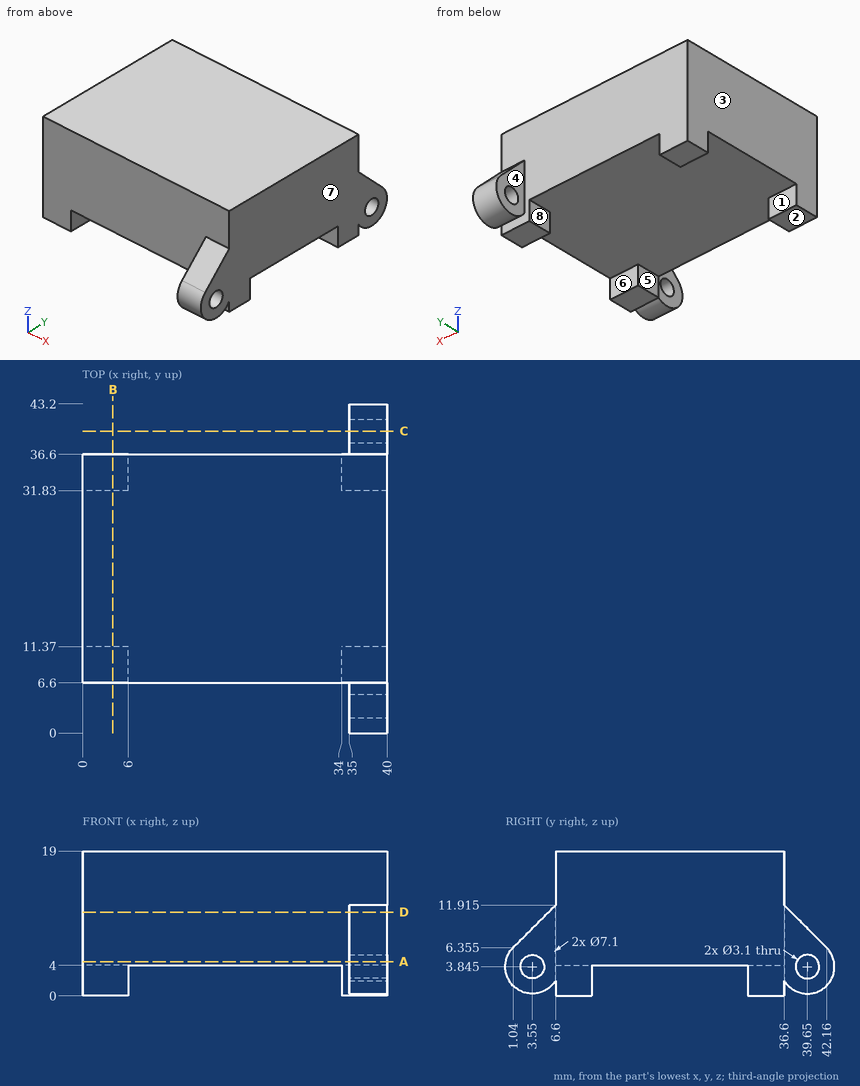
Geometry: see drawing. Coordinates: mm, zero at the bounding-box minimum. A direction names the side the tool comes from. Coordinates: 2 decimals unless noted, no trailing zeros. Write each loop counter-clockwise with the first axis right and the second up, starting at its lowest first coordinate (ties: lowest second). Pieces come first, ordered by that corner, then holes.
1) Pin query (flat end, axial travel): pin 1 Ø9.5 at (x, z) = (23.5, 8) entering from -Y; pin 2 Ø3.5 at (y, z) = (4.5, 6) entering from -X; pin 3 Ø6 at (x, y) = (25.5, 19.5) entering from -Z. Return the tip coordinate at first contact, or that it passes through.
2) Material intervals for line 1 along X through (y, z) = (35.5, 3.25); line 2 along Y through (x, z) = (3, 1.5); line 3 along Z through (x, y) = (34.5, 27), sorted ascending.
3) Set-up query: the marked faces 1, 2, 3, 4 and 5. Return all of +Z, -Z, +X, -X, +Y, -Y with unobstructed straight access to the full face (end or side cutting, diameter ignored); none if empty.
4) Section C-C on y = 39.65. Output: boundary loops of the cut face in (x, z) (1 decimal).
5) Section B-B on x = 4. Output: boundary loops of the cut face in (y, z), and give its area (3 significant figures).
6) Mould query, pull axis X, two halves, no side actions, for the marked faces 6, 7 and 8. Classes: pulls with the +X half, pulls with the -X half, needs draft (parallel to the pull), parting line crosses it, or undercut.
7) Section A-A on z = 4.5. Output: boundary loops of the cut face in (x, y) (1 decimal).
8) Section D-D on z = 11. Output: boundary loops of the cut face in (x, y) (1 decimal).
Check result:
1. pin 1: stops at y = 6.6
1. pin 2: stops at x = 35
1. pin 3: stops at z = 4
2. line 1: x = 0 to 6, 34 to 40
2. line 2: y = 6.6 to 11.37, 31.83 to 36.6
2. line 3: z = 4 to 19
3. face 1: -Z, +X, -X
3. face 2: -Z, +X, -X, +Y, -Y
3. face 3: +Z, -Z, -X, +Y, -Y
3. face 4: +Z, -Z, -X, +Y
3. face 5: -Z, +Y, -Y
4. outline: (35, 0.3) - (40, 0.3) - (40, 2.3) - (35, 2.3) - close; (35, 5.4) - (40, 5.4) - (40, 8.9) - (35, 8.9) - close
5. outline: (6.6, 0) - (11.37, 0) - (11.37, 4) - (31.83, 4) - (31.83, 0) - (36.6, 0) - (36.6, 19) - (6.6, 19) - close
5. area: 488 mm2
6. face 6: needs draft
6. face 7: pulls with the +X half
6. face 8: undercut
7. outline: (0, 6.6) - (35, 6.6) - (35, 5) - (40, 5) - (40, 38.2) - (35, 38.2) - (35, 36.6) - (0, 36.6) - close; (35, 0.1) - (40, 0.1) - (40, 2.1) - (35, 2.1) - close; (35, 41.1) - (40, 41.1) - (40, 43.1) - (35, 43.1) - close
8. outline: (0, 6.6) - (35, 6.6) - (35, 5.7) - (40, 5.7) - (40, 37.5) - (35, 37.5) - (35, 36.6) - (0, 36.6) - close
